```python
from build123d import *

# Parameters (mm, degrees)
SKETCH1_W                  = 80.3
SKETCH1_H                  = 66
BOSS_EXTRUDE1_DEPTH        = 3
F_3_2_3_2_DIAMETER_HOLE1_D = 3.2
SKETCH2_W                  = 57.29
SKETCH2_H                  = 38.19
CUT_EXTRUDE1_DEPTH         = 4
FILLET1_R                  = 3.5
FILLET2_R                  = 2.5


with BuildPart() as part:
    # Sketch1 → Boss-Extrude1 (new body)
    with BuildSketch(Plane.XY):
        with Locations((40.15, 33)):
            Rectangle(SKETCH1_W, SKETCH1_H)
    extrude(amount=BOSS_EXTRUDE1_DEPTH)

    # Ø3.2 (3.2) Diameter Hole1 (through all)
    with Locations(Plane.XY.offset(3)):
        with Locations((7, 59), (73.3, 59), (73.3, 7), (7, 7)):
            Hole(F_3_2_3_2_DIAMETER_HOLE1_D / 2)

    # Sketch2 → Cut-Extrude1 (cut, through all)
    with BuildSketch(Plane.XY.offset(3)):
        with Locations((42.935, 32.995)):
            Rectangle(SKETCH2_W, SKETCH2_H)
    extrude(amount=-CUT_EXTRUDE1_DEPTH, mode=Mode.SUBTRACT)

    # Fillet1
    fillet1_edges = [part.edges().sort_by_distance(p)[0] for p in [
        (0, 66, 1.5),
        (80.3, 66, 1.5),
        (80.3, 0, 1.5),
        (0, 0, 1.5),
    ]]
    fillet(fillet1_edges, radius=FILLET1_R)

    # Fillet2
    fillet2_edges = [part.edges().sort_by_distance(p)[0] for p in [
        (14.29, 13.9, 1.5),
        (14.29, 52.09, 1.5),
        (71.58, 52.09, 1.5),
        (71.58, 13.9, 1.5),
    ]]
    fillet(fillet2_edges, radius=FILLET2_R)


solid = part.part
```
The listing builds one solid part. Answer for the finished solid, in the listing's coordinates (mm). A direction names the side the tool comes from. Round coordinates to 2 decimals unless told otherwise and drop trailing zeros. Loops run counter-clockwise (first coordinate to the right, second up) from the corner with the lowest first, then second, coordinate; pieces in that order, holes last.
1) For faces 1 (the face through (79.25, 1, 1.52)), 2 (the face through (43, 52.09, 2)), determine the directions among +Z, -Z, +X, -X, +Y, -Y from which every point of the face is accessible in a straight line to the end or side of a thin tool.
Outcome:
face 1: +Z, -Z, +X, -Y
face 2: +Z, -Z
2) A cutting plane is placed at A-A on y = 7. Determine the outline of the cut face in (x, z).
Outcome:
outline: (0, 0) - (5.4, 0) - (5.4, 3) - (0, 3) - close; (8.6, 0) - (71.7, 0) - (71.7, 3) - (8.6, 3) - close; (74.9, 0) - (80.3, 0) - (80.3, 3) - (74.9, 3) - close
3) A cutting plane is placed at C-C on z = 1.8. Determine the outline of the cut face in (x, y).
Outcome:
outline: (0, 3.5) arc R3.5 ccw to (3.5, 0) - (76.8, 0) arc R3.5 ccw to (80.3, 3.5) - (80.3, 62.5) arc R3.5 ccw to (76.8, 66) - (3.5, 66) arc R3.5 ccw to (0, 62.5) - close; hole circle Ø3.2 at (7, 7); hole circle Ø3.2 at (7, 59); hole (14.29, 16.4) arc R2.5 ccw to (16.79, 13.9) - (69.08, 13.9) arc R2.5 ccw to (71.58, 16.4) - (71.58, 49.59) arc R2.5 ccw to (69.08, 52.09) - (16.79, 52.09) arc R2.5 ccw to (14.29, 49.59) - close; hole circle Ø3.2 at (73.3, 7); hole circle Ø3.2 at (73.3, 59)
4) For a pull along Y with two mould halves and no side action, classify faces 3 (the face through (70.867, 51.338, 1.479)), 4 (the face through (74.9, 7.07, 1.48)), 5 (the face through (0, 33, 1)), 6 (the face through (40, 66, 1)) as released by +Y, released by -Y, zero draft, split by the parting line, or undercut.
Outcome:
face 3: undercut
face 4: undercut
face 5: zero draft
face 6: released by +Y
5) A cutting plane is placed at B-B on x = 73.3. Determine the outline of the cut face in (y, z).
Outcome:
outline: (0, 0) - (5.4, 0) - (5.4, 3) - (0, 3) - close; (8.6, 0) - (57.4, 0) - (57.4, 3) - (8.6, 3) - close; (60.6, 0) - (66, 0) - (66, 3) - (60.6, 3) - close
6) A cutting plane is placed at D-D on x = 44. Determine the outline of the cut face in (y, z).
Outcome:
outline: (0, 0) - (13.9, 0) - (13.9, 3) - (0, 3) - close; (52.09, 0) - (66, 0) - (66, 3) - (52.09, 3) - close
7) Consider line 1 (Y direction, x = 73.3, z = 2); line 2 (Y direction, x = 68, z = 1.15); line 3 (X direction, y = 40.5, z = 0.4). Determine where each line is inside the solid, lowest interval first.
Outcome:
line 1: y = 0 to 5.4, 8.6 to 57.4, 60.6 to 66
line 2: y = 0 to 13.9, 52.09 to 66
line 3: x = 0 to 14.29, 71.58 to 80.3
